Solid Edge part; units mm, degrees
sketch "Sketch1" plane through (0, 0, 0) normal (0, 0, 1) x (1, 0, 0)
  line L0 (-10, -10) -> (10, -10)
  line L1 (10, -10) -> (10, 10)
  line L2 (10, 10) -> (-10, 10)
  line L3 (-10, 10) -> (-10, 2.65)
  line L4 (-8.5, 2.65) -> (-10, 2.65)
  line L5 (-8.5, 4.25) -> (-8.5, 2.65)
  line L6 (-3.3, 4.25) -> (-8.5, 4.25)
  arc A0 (-3.3, 4.25) -> (-3.3, -4.25) centre (-8.5833, 0) cw
  line L7 (-8.5, -4.25) -> (-3.3, -4.25)
  line L8 (-8.5, -2.65) -> (-8.5, -4.25)
  line L9 (-10, -2.65) -> (-8.5, -2.65)
  line L10 (-10, -2.65) -> (-10, -10)
extrude "Protrusion1" add sketch "Sketch1" along normal blind 61
sketch "Sketch2" plane through (0, 10, 30.5) normal (0, 1, 0) x (-1, 0, 0)
  line L0 (-10, 30.5) -> (-10, 10.5)
  line L1 (-10, 10.5) -> (-5, 10.5)
  line L2 (-5, 10.5) -> (-5, 30.5)
  line L3 (-5, 30.5) -> (-10, 30.5)
extrude "Protrusion2" add sketch "Sketch2" along normal blind 20
sketch "Sketch3" plane through (0, 10, 30.5) normal (0, 1, 0) x (-1, 0, 0)
  line L0 (-5, 10.5) -> (-5, 30.5)
  line L1 (-5, 30.5) -> (-10, 30.5)
  line L2 (-10, 30.5) -> (-10, 10.5)
  line L3 (-10, 10.5) -> (-5, 10.5)
extrude "Protrusion3" add sketch "Sketch3" against normal blind 40
Check sheet for the modelled part. Datum: model origin and axes. Units: mm. A direction names the side the tool comes from. Round coordinates to 2 decimals unless told otherwise and drop trailing zeros. Loops run counter-clockwise (first coordinate to the right, second up) from the corner with the lowest first, then second, coordinate; pieces in that order, holes last. Notation, with made-up numbers: (-17.5, 7.25) -> (36.5, 7.25) arc R24 cw to (36.5, 24.25) -> close; hole circle Ø1 at (-24.5, -28). An arc over 180 degrees is marked (long way). Write item = value, one per line. Start each with the question number.
1) Gauge pin test, flat ends, axial feed: pin 1 Ø1 at (x, z) = (5.5, 34.5) entering from -Y; pin 2 Ø3 at (x, z) = (-4.5, 8.5) entering from +Y; pin 3 Ø22 at (y, z) = (24.5, 55) entering from -X; pin 4 Ø16 at (y, z) = (-16.5, 51.5) entering from -X. Record the tip position at first contact, or that the pin passes through.
2) Sectioned sample at A-A, the plane x = -4.25. Record the cut outline in (y, z), plus the area to 4 significant figures.
3) Thickness scan on probe 1 along Y at (x, z) = (-9, 10); probe 2 along Y at (x, z) = (-0.75, 20); probe 3 along X at (y, z) = (19.5, 57.5). Record the ranges inside material, lowest first.
4) Sectioned sample at D-D, the plane y = -17.5. Record the cut outline in (x, z), plus the area to 3 significant figures.
5) Sectioned sample at B-B, the plane z = 50. Record the cut outline in (x, y), plus the area to 3 significant figures.
6) Set-up check for faces 4 (the flat face through (5, 20, 51)), 5 (the cylindrical face through (-1.803, 0.064, 30.073)), 6 (the flat face through (-9, -2.65, 30)), 7 (the flat face through (8, 20, 41)): record each of +Z, -Z, +X, -X, +Y, -Y from which the full face is reachable in a straight line by a thin tool's end or side.
7) Sectioned sample at C-C, the plane x = 5.75. Record the cut outline in (y, z), plus the area to 3 significant figures.
8) Release check for a two-part mould opening along Y. For faces 1 (the flat face through (5, -20, 51)), 2 (the flat face through (8, 30, 51)), 3 (the flat face through (-6, 4.25, 30)) record: released by +Y, released by -Y, zero draft, split by the parting line, or undercut.
Results are:
q1.pin_1 = -10
q1.pin_2 = 10
q1.pin_3 = 5
q1.pin_4 = -10
q2.outline = (-10, 0) -> (-4.25, 0) -> (-4.25, 61) -> (-10, 61) -> close; (4.25, 0) -> (10, 0) -> (10, 61) -> (4.25, 61) -> close
q2.area = 701.5 mm^2
q3.probe_1 = -10 to -2.65, 2.65 to 10
q3.probe_2 = -10 to 10
q3.probe_3 = 5 to 10
q4.outline = (5, 41) -> (10, 41) -> (10, 61) -> (5, 61) -> close
q4.area = 100 mm^2
q5.outline = (-10, -10) -> (5, -10) -> (5, -30) -> (10, -30) -> (10, 30) -> (5, 30) -> (5, 10) -> (-10, 10) -> (-10, 2.65) -> (-8.5, 2.65) -> (-8.5, 4.25) -> (-3.3, 4.25) arc R6.78 cw to (-3.3, -4.25) -> (-8.5, -4.25) -> (-8.5, -2.65) -> (-10, -2.65) -> close
q5.area = 539 mm^2
q6.face_4 = +Z, -Z, -X, +Y
q6.face_5 = +Z, -Z
q6.face_6 = +Z, -Z, -X
q6.face_7 = -Z, +X, -X, +Y
q7.outline = (-30, 41) -> (-10, 41) -> (-10, 0) -> (10, 0) -> (10, 41) -> (30, 41) -> (30, 61) -> (-30, 61) -> close
q7.area = 2,020 mm^2
q8.face_1 = zero draft
q8.face_2 = released by +Y
q8.face_3 = undercut
